The listing builds one solid part. Answer for the finished solid, in the listing's coordinates (mm). A direction names the side the tool comes from. Give positions to 0.01 mm unless a question says otherwise; leave off trailing zeros. Loops run counter-clockwise (first coordinate to the right, second up) from the corner with the lowest first, then second, coordinate; pieces in that order, holes last.
Item 1: Section B-B, the plane y = -2.5 is taken. Give the vertices of the cut face in (x, z) (3 decimals), and give its area (3 significant figures).
Item 2: The mould has two halves that part along Z. Classify faces 4 (the face through (15, 2.8, -1)), 5 (the face through (-0.729, -2.958, 3.285)), 6 (the face through (16.63, 1.38, -5.22)): pulls with the +Z half, pulls with the -Z half, needs draft (parallel to the pull), parting line crosses it, or undercut.
Item 3: Section A-A, the plane x = 0 is taken. Give the vertices of the cut face in (y, z) (3 decimals), and give its area (3 significant figures).
Item 4: Each of these flat-tipped pins is pushed along its axis until it touches: pin 1 Ø3.5 at (x, z) = (-0.5, -0.5) entering from -Y; pin 2 Ø2.5 at (x, z) = (0, 0) entering from -Y; pin 3 Ø4 at (x, y) = (22.5, -1) entering from +Z. Where does it stop, or does it pass through?
Item 5: A tool of negligible diameter and unlimited length cuts with its end or side. For faces 1 (the face through (9.6, 1.4, 0)), 2 (the face through (0.7, 2.24, -1.5)), 3 (the face through (0, 0, 2)), from which of +Z, -Z, +X, -X, +Y, -Y can it reach the whole face along a straight path? Write none if from no direction.
Item 6: Section D-D, the plane x = 14 is taken. Give the vertices of the cut face in (y, z).
Item 7: Section C-C, the plane z = 0 is taken. Give the number of separate pieces and of enclosed holes in the cut face, and give its area (3 significant figures).
Item 8: Consider line 1 along X through (y, z) = (-4.5, -0.5); line 2 along Y through (x, z) = (9, -3); line 3 along X through (y, z) = (-1.5, 1.5). Determine where each line is inside the solid, lowest interval first.
Autodesk Inventor part; units mm, degrees
ref_plane "YZ Plane" through (0, 0, 0) normal (1, 0, 0) x (0, 1, 0)
ref_plane "XZ Plane" through (0, 0, 0) normal (0, 1, 0) x (-1, 0, 0)
ref_plane "XY Plane" through (0, 0, 0) normal (0, 0, 1) x (1, 0, 0)
sketch "Sketch1" plane through (0, 0, 0) normal (0, 1, 0) x (-1, 0, 0)
  arc A0 (-0.5058, -6.4803) -> (-0.5058, 6.4803) centre (0, 0) ccw
  arc A1 (-32.3013, 3.9986) -> (-32.3013, -3.9986) centre (-31.9892, 0) ccw
  line L0 (-32.3013, -3.9986) -> (-0.5058, -6.4803)
  line L1 (-0.5058, 6.4803) -> (-32.3013, 3.9986)
  circle A2 centre (0, 0) radius 1.47
  circle A3 centre (-14, 0) radius 1
  circle A4 centre (-19.4, 0) radius 1
  circle A5 centre (-24.8, 0) radius 1
  circle A6 centre (-30.2, 0) radius 1
  circle A7 centre (-8.6, 0) radius 1
  point P0 (-36, 0)
  point P1 (-36, 0)
  dimension "d0" = 0
  dimension "d1" = 0
  dimension "d2" = 13
  dimension "d3" = 0
  dimension "d4" = 42.5
  dimension "d5" = 2.94
  dimension "d6" = 5.4
  dimension "d7" = 5.4
  dimension "d8" = 5.4
  dimension "d9" = 5.4
  dimension "d10" = 0
  dimension "d11" = 5.8
  dimension "d12" = 2
  dimension "d13" = 2
  dimension "d14" = 2
  dimension "d15" = 2
  dimension "d16" = 2
  dimension "d17" = 0
  dimension "d18" = 0
  dimension "d19" = 0
  dimension "d20" = 0
  dimension "d21" = 0
  dimension "d22" = 3.15
extrude "Extrusion1" add sketch "Sketch1" along normal blind 2.8
sketch "Sketch2" plane through (0, 0, 0) normal (0, -1, 0) x (1, 0, 0)
  circle A0 centre (0, 0) radius 3.365 construction
  arc A1 (0.5058, 6.4803) -> (0.5058, -6.4803) centre (0, 0) ccw
  circle A2 centre (0, 0) radius 5.515
  circle A3 centre (0, 0) radius 3.365
  dimension "d25" = 11.03
  dimension "d28" = 6.73
extrude "Extrusion3" add sketch "Sketch2" along normal blind 6
sketch "Sketch3" plane through (0, 2.8, 0) normal (0, 1, 0) x (1, 0, 0)
  circle A0 centre (0, 0) radius 1.47
  arc A1 (0.5058, 6.4803) -> (0.5058, -6.4803) centre (0, 0) ccw
  circle A2 centre (0, 0) radius 3.2
  dimension "d31" = 6.4
extrude "Extrusion4" cut sketch "Sketch3" against normal blind 0.56
equation "\"d7\" = d6"
equation "\"d8\" = d6"
equation "\"d9\" = d6"
equation "\"d13\" = d12"
equation "\"d14\" = d12"
equation "\"d15\" = d12"
equation "\"d16\" = d12"
properties part number "ServoHorn"
Worked answers:
1. outline: circle Ø11.03 at (0, 0); hole circle Ø6.73 at (0, 0)
1. area: 60.0 mm2
2. face 4: needs draft
2. face 5: undercut
2. face 6: pulls with the -Z half
3. outline: (-6, -5.515) - (0, -5.515) - (0, -6.5) - (2.8, -6.5) - (2.8, -3.2) - (2.24, -3.2) - (2.24, -1.47) - (0, -1.47) - (0, -3.365) - (-6, -3.365) - close; (-6, 3.365) - (0, 3.365) - (0, 1.47) - (2.24, 1.47) - (2.24, 3.2) - (2.8, 3.2) - (2.8, 6.5) - (0, 6.5) - (0, 5.515) - (-6, 5.515) - close
3. area: 52.0 mm2
4. pin 1: stops at y = 0
4. pin 2: passes through
4. pin 3: stops at z = 4.9
5. face 1: +Y, -Y
5. face 2: +Y
5. face 3: -Y
6. outline: (0, -5.43) - (2.8, -5.43) - (2.8, -1) - (0, -1) - close; (0, 1) - (2.8, 1) - (2.8, 5.43) - (0, 5.43) - close
7. separate pieces: 7
7. enclosed holes: 0
7. area: 107 mm2
8. line 1: x = -5.49 to -3.33, 3.33 to 5.49
8. line 2: y = 0 to 2.8
8. line 3: x = -5.31 to -3.01, 3.01 to 5.31
